Autodesk Fusion 360 part; units mm, degrees
sketch "Skizze1" plane through (0, 0, 0) normal (0, 0, 1) x (1, 0, 0)
  line L0 (10, 10) -> (13, 10)
  line L1 (13, 10) -> (13, 23)
  line L2 (13, 23) -> (10, 23)
  line L3 (10, 23) -> (10, 10)
  line L4 (10, 23) -> (90, 23)
  line L5 (90, 23) -> (90, 26)
  line L6 (90, 26) -> (10, 26)
  line L7 (10, 26) -> (10, 23)
  line L8 (14, 26) -> (17, 26)
  line L9 (15.5, 26) -> (15.5, 41)
  line L10 (15.5, 41) -> (16.5, 41)
  line L11 (15.5, 41) -> (14.5, 41)
  line L12 (14.5, 41) -> (14, 26)
  line L13 (16.5, 41) -> (17, 26)
  dimension "d1" = 3
  dimension "d2" = 13
  dimension "d3" = 80
  dimension "d4" = 3
  dimension "d5" = 3
  dimension "d6" = 15
  dimension "d7" = 1
  dimension "d8" = 1
extrude "Extrusion1" add sketch "Skizze1" along normal blind 50
sketch "Skizze2" plane through (13, 0, 0) normal (1, 0, 0) x (0, 1, 0)
  line L0 (10, 0) -> (23, 0)
  line L1 (23, 0) -> (23, 50)
  line L2 (23, 50) -> (10, 50)
  line L3 (10, 50) -> (10, 0)
  circle A0 centre (16, 45) radius 1.5
  circle A1 centre (16, 5) radius 1.5
  dimension "d11" = 3
  dimension "d12" = 3
extrude "Extrusion2" cut sketch "Skizze2" against normal blind 3 contours A0 | A1
sketch "Skizze3" plane through (0, 23, 0) normal (0, -1, 0) x (1, 0, 0)
  line L0 (13, 0) -> (90, 0)
  line L1 (90, 0) -> (90, 50)
  line L2 (90, 50) -> (13, 50)
  line L3 (13, 50) -> (13, 0)
  line L4 (90, 23) -> (13, 23)
  line L5 (13, 23) -> (13, 27)
  line L6 (13, 27) -> (90, 27)
  line L7 (90, 27) -> (90, 23)
  line L8 (90, 23) -> (13, 27) construction
  line L9 (13, 23) -> (90, 27) construction
  dimension "d15" = 4
extrude "Extrusion3" add sketch "Skizze3" along normal blind 3 contours L1 L3 L4 L5 L6 L7
chamfer "Fase1" distance 3 angle 45 1 edges at (51.5, 23, 27)
chamfer "Fase2" distance 3 angle 45 1 edges at (51.5, 23, 23)
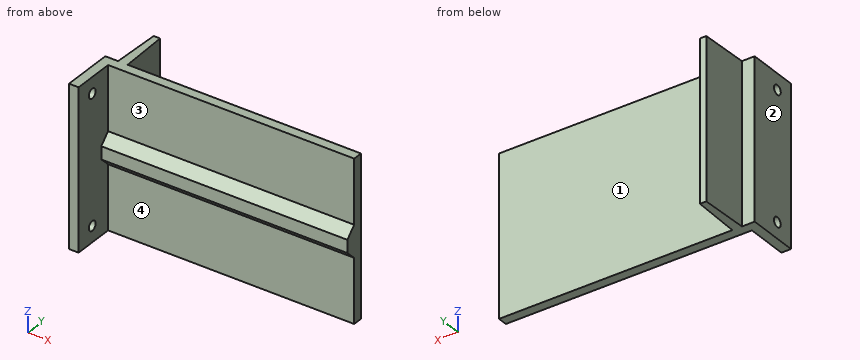
Geometry check sheet. Reference: the model listing, model coordinates, mm. Face numbers are marked on the shaded views. A direction names the side the tool comes from. Give positions to 0.01 mm unless a question says otherwise; leave off trailing zeros. Order: outer loops, then holes, each group sorted by start corner. A loop starts at its lowest first (then second) coordinate and runs counter-clockwise, first axis right, second up. Notation, with made-up numbers: (27.5, 41.5) -> (67.5, 41.5) arc R23 ccw to (67.5, 66.5) -> close; hole circle Ø9 at (-35.5, -28). An arc over 180 degrees is marked (long way). Write each question's results on one line, items separated by ' | '. Start each with the question number.
(1) Gauge pin test, flat ends, axial feed: P1, Ø1.2, axis at x = 43.5, z = 25.5, coming from the -Y side; P2, Ø2, axis at x = 12.5, z = 22.5, coming from the +Y side; P3, Ø2, axis at x = 49.5, z = 35.5, coming from the -Y side; P4, Ø8, axis at x = 69.5, y = 15, coming from the +Z side. Record the tip position at first contact, or that the pin passes through.
(2) Access from +Z, -Z, +X, -X, +Y, -Y to the whole of each face (thin tool, end or side, straight path). Record for the marked faces 1, 2, 3 and 4.
(3) Sectioned sample at D-D (z = 17.5). Enter the section's corners in (x, y).
(4) Sectioned sample at B-B (z = 45). Enter the section's corners in (x, y).
(5) Sectioned sample at A-A (y = 16). Enter the section's corners in (x, z), plus the area to 3 significant figures.
(6) Scan lines: line 1 (Z direction, x = 11.25, y = 16); line 2 (X direction, y = 19, z = 4); line 3 (Y direction, x = 75.5, z = 45.5). Record each from-to range of solid material in increasing order.
Answer below:
1) P1: y = 20 | P2: y = 26 | P3: y = 23 | P4: through
2) face 1: +Z, -Z, +X, +Y | face 2: +Z, -Z, -X, +Y, -Y | face 3: +Z, +X, -Y | face 4: -Z, +X, -Y
3) outline: (10, 10) -> (13, 10) -> (13, 23) -> (90, 23) -> (90, 26) -> (17, 26) -> (16.5, 41) -> (14.5, 41) -> (14, 26) -> (10, 26) -> close
4) outline: (10, 10) -> (13, 10) -> (13, 14.5) -> (10, 14.5) -> close; (10, 17.5) -> (13, 17.5) -> (13, 23) -> (90, 23) -> (90, 26) -> (17, 26) -> (16.5, 41) -> (14.5, 41) -> (14, 26) -> (10, 26) -> close
5) outline: (10, 0) -> (13, 0) -> (13, 3.5) -> (10, 3.5) -> close; (10, 6.5) -> (13, 6.5) -> (13, 43.5) -> (10, 43.5) -> close; (10, 46.5) -> (13, 46.5) -> (13, 50) -> (10, 50) -> close | area: 132 mm2
6) line 1: 0 to 3.5, 6.5 to 43.5, 46.5 to 50 | line 2: 10 to 13 | line 3: 23 to 26
